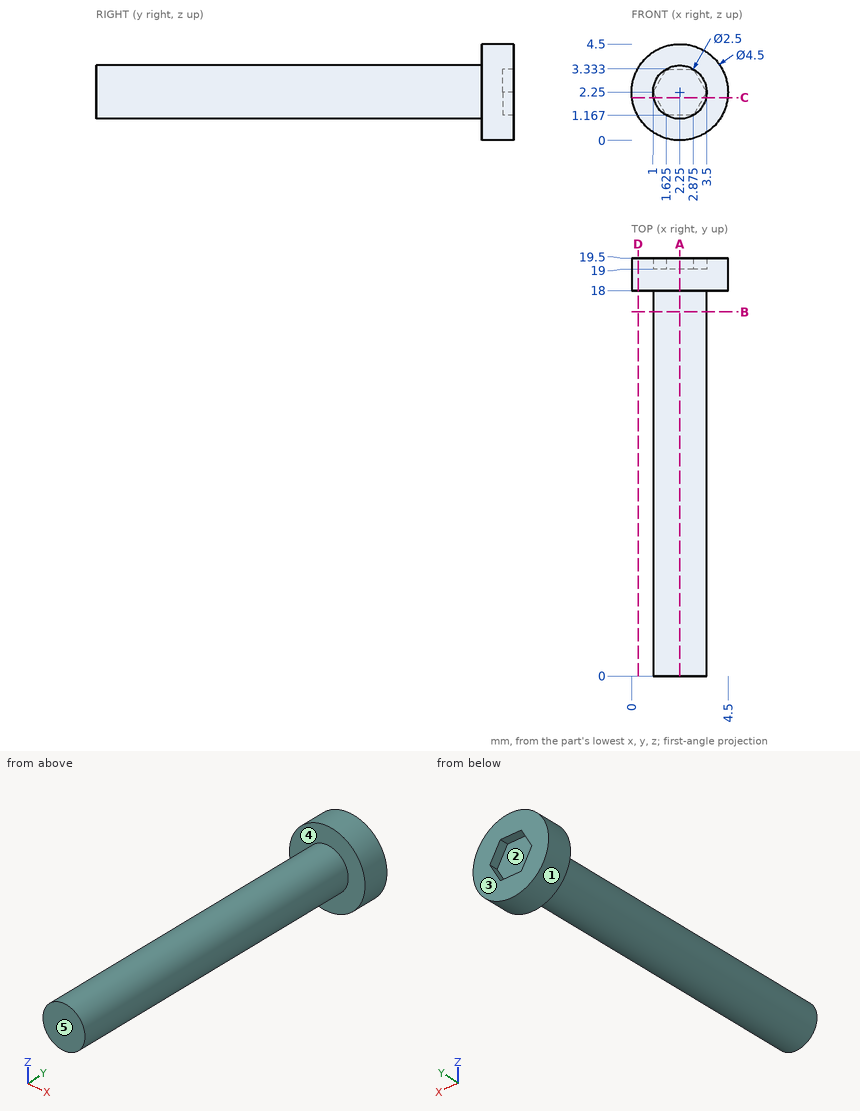
Study the drawing (mm; zero at the part's minimum x, y, z) and answer. A direction names the side the tool comes from. Give positions to 0.01 mm unless a question says otherwise; leave off trailing zeros. Order: outer loops, then holes, each group sorted by start corner. A loop starts at its lowest first (then second) coordinate and runs counter-clockwise, first axis right, second up. Notation, with made-up numbers: (-34, 48) - (-14, 48) arc R24 ccw to (-14, 78) - close; hole circle Ø11 at (-19.75, 15). An arc over 180 degrees is marked (long way). Use one line per item in the form item = value. Start each with the question number.
(1) The mould has two halves that part along Z. Classify the marked faces 1, 2 and 3: released by +Z, released by -Z, zero draft, split by the parting line, or undercut.
(2) A cutting plane is placed at D-D, the plane x = 0.3. Write down the section's boundary in (y, z).
(3) For the marked faces 4 and 5, determine the directions among +Z, -Z, +X, -X, +Y, -Y from which every point of the face is accessible in a straight line to the end or side of a thin tool.
(4) Flat-ended cylindrical pins translate along their axes: pin 1 Ø1.5 at (x, y) = (1.5, 10.5) entering from -Z; pin 2 Ø1 at (x, y) = (2, 7) entering from +Z; pin 3 Ø2 at (y, z) = (8, 2) entering from -X. Find the tip coordinate at first contact, or state that the pin passes through.
(5) A cutting plane is placed at C-C, the plane z = 2. Write down the section's boundary in (x, y) (1 decimal).
(6) A cutting plane is placed at A-A, the plane x = 2.25. Write down the section's boundary in (y, z).
(7) A cutting plane is placed at B-B, the plane y = 17. Write down the section's boundary in (x, z).
(8) Consider line 1 (Y direction, x = 3.3, z = 0.55); line 2 (Y direction, x = 2, z = 3.1); line 3 (X direction, y = 4, z = 2.2). Determine where each line is inside the solid, lowest interval first. Write a range as from..to.
Ans:
q1.face_1 = split by the parting line
q1.face_2 = undercut
q1.face_3 = zero draft
q2.outline = (18, 1.13) - (19.5, 1.13) - (19.5, 3.37) - (18, 3.37) - close
q3.face_4 = -Y
q3.face_5 = +Z, -Z, +X, -X, -Y
q4.pin_1 = 1
q4.pin_2 = 3.5
q4.pin_3 = 1
q5.outline = (0, 18) - (1, 18) - (1, 0) - (3.5, 0) - (3.5, 18) - (4.5, 18) - (4.5, 19.5) - (3.4, 19.5) - (3.4, 19) - (1.1, 19) - (1.1, 19.5) - (0, 19.5) - close
q6.outline = (0, 1) - (18, 1) - (18, 0) - (19.5, 0) - (19.5, 1.17) - (19, 1.17) - (19, 3.33) - (19.5, 3.33) - (19.5, 4.5) - (18, 4.5) - (18, 3.5) - (0, 3.5) - close
q7.outline = circle Ø2.5 at (2.25, 2.25)
q8.line_1 = 18..19.5
q8.line_2 = 0..19
q8.line_3 = 1..3.5
